Design review of the part built by this model. Coordinates are the model's own, in mm. Face numbers are marked on the shaded views. A direction names the side the tool comes from. Coordinates: 2 decimals unless noted, no trailing zeros. Loops run counter-clockwise (first coordinate to the right, second up) from the corner with the lowest first, then second, coordinate; pieces in that order, holes last. Notation, with made-up numbers: M -36,70 L -4,70 A21 cw -4,101 Z; hole C 28.25,-23 d3. An arc over 180 degrees is marked long. Answer as a JSON object with one key per item and string values. Group by question number.
1. Consider section C-C (y = 22). State the section outline as (x, z) points, then the cut area to 3 significant figures.
2. Consider section A-A (z = 0). State the section outline as (x, y) points, then the cut area to 3 significant figures.
3. To check wall thickness, follow probe 1 along Z at (x, y) = (-7, 5.5); probe 2 along X at (y, z) = (3, -2.5); probe 3 along X at (y, z) = (1.5, 0). State the ranges of each line that lie inside material, in increasing order.
4. Consider section B-B (x = 0). State the section outline as (y, z) points.
5. Insertion check: pin 1 (18 mm diameter, centred on x = -7.5, z = 3.5, fed in from +Y). The pin has a flat end and moves straight along its axis. Give the tip position at first contact, or say it passes through.
6. Draft analysis for pull direction X (two halves, no side actions). For the marked faces 3, 4, 5 and 6, state which applies: +X half, -X half, draft (parallel to the pull), parting line (faces both ways), or undercut.
7. Machinability: for the marked faces 1 and 2, which of the approach directions +Z, -Z, +X, -X, +Y, -Y give a long, thin tool a straight path to every point of the face, cutting with its end or side? Answer none if there is none.
8. Consider section D-D (z = -10.5). State the section outline as (x, y) points.
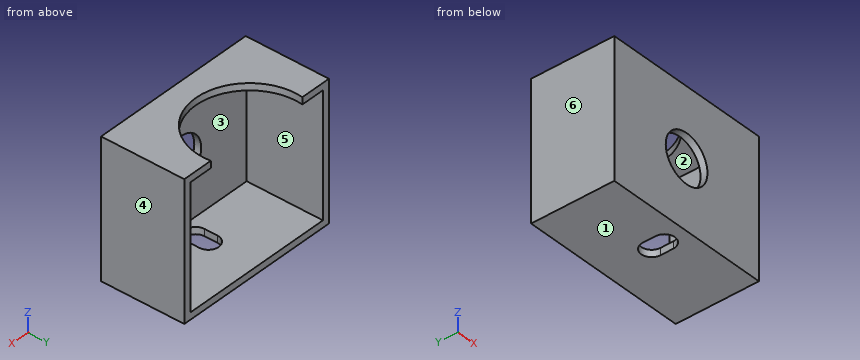
from build123d import *

# Parameters (mm, degrees)
SKETCH_2_W          = 48.5
SKETCH_2_H          = 39.5
EXTRUDE_1_DEPTH     = 2
SKETCH_4_W          = 48.5
SKETCH_4_H          = 39.5
SKETCH_4_W_2        = 44.5
SKETCH_4_H_2        = 35.5
EXTRUDE_2_DEPTH     = 22
SKETCH_5_R          = 15.5
CUT_EXTRUDE_1_DEPTH = 10
CUT_EXTRUDE_2_DEPTH = 10
SKETCH_7_R          = 7
CUT_EXTRUDE_3_DEPTH = 10


with BuildPart() as part:
    # 草图2 → 凸台-拉伸1 (new body)
    with BuildSketch(Plane(origin=(0, 0, 0), x_dir=(1, 0, 0), z_dir=(0, 1, 0))):
        Rectangle(SKETCH_2_W, SKETCH_2_H)
    extrude(amount=EXTRUDE_1_DEPTH)

    # 草图4 → 凸台-拉伸2 (add)
    with BuildSketch(Plane(origin=(0, 2, 0), x_dir=(1, 0, 0), z_dir=(0, 1, 0))):
        Rectangle(SKETCH_4_W, SKETCH_4_H)
        Rectangle(SKETCH_4_W_2, SKETCH_4_H_2, mode=Mode.SUBTRACT)
    extrude(amount=EXTRUDE_2_DEPTH)

    # 草图5 → 切除-拉伸1 (cut)
    with BuildSketch(Plane.XY.offset(19.75)):
        with Locations((0, 22)):
            Circle(SKETCH_5_R)
    extrude(amount=-CUT_EXTRUDE_1_DEPTH, mode=Mode.SUBTRACT)

    # 草图6 → 切除-拉伸2 (cut)
    with BuildSketch(Plane(origin=(0, 0, -19.75), x_dir=(-1, 0, 0), z_dir=(0, 0, -1))):
        with BuildLine():
            Line((3, 10.070876888), (3, 6.403632954))
            ThreePointArc((3, 6.403632954), (0, 3.403632954), (-3, 6.403632954))
            Line((-3, 6.403632954), (-3, 10.070876888))
            ThreePointArc((-3, 10.070876888), (0, 13.070876888), (3, 10.070876888))
        make_face()
    extrude(amount=-CUT_EXTRUDE_2_DEPTH, mode=Mode.SUBTRACT)

    # 草图7 → 切除-拉伸3 (cut)
    with BuildSketch(Plane.XZ):
        with Locations(Location((0, 0, 0), (0, 0, 270))):
            Circle(SKETCH_7_R)
    extrude(amount=-CUT_EXTRUDE_3_DEPTH, mode=Mode.SUBTRACT)


solid = part.part
Findings below:
{
 "1": {"outline": "M -24.25,-19.75 L 24.25,-19.75 L 24.25,19.75 L 15.5,19.75 L 15.5,17.75 L 22.25,17.75 L 22.25,-17.75 L -22.25,-17.75 L -22.25,17.75 L -15.5,17.75 L -15.5,19.75 L -24.25,19.75 Z", "area": "274 mm^2"},
 "2": {"outline": "M -24.25,0 L -7,0 L -7,2 L -22.25,2 L -22.25,24 L -24.25,24 Z; M 7,0 L 24.25,0 L 24.25,24 L 22.25,24 L 22.25,2 L 7,2 Z", "area": "157 mm^2"},
 "3": {"probe 1": "z = -19.75 to -17.75, 17.75 to 19.75", "probe 2": "x = -24.25 to -22.25, 22.25 to 24.25", "probe 3": "x = -24.25 to -7, 7 to 24.25"},
 "4": {"outline": "M 0,-19.75 L 3.4,-19.75 L 3.4,-17.75 L 2,-17.75 L 2,-7 L 0,-7 Z; M 0,7 L 2,7 L 2,17.75 L 6.5,17.75 L 6.5,19.75 L 0,19.75 Z; M 13.07,-19.75 L 24,-19.75 L 24,-17.75 L 13.07,-17.75 Z"},
 "5": {"pin 1": "stops at y = 2"},
 "6": {"face 3": "undercut", "face 4": "+X half", "face 5": "undercut", "face 6": "-X half"},
 "7": {"face 1": "-Z, +X, -X, +Y, -Y", "face 2": "+Y"},
 "8": {"outline": "M -24.25,0 L 24.25,0 L 24.25,24 L 22.25,24 L 22.25,2 L -22.25,2 L -22.25,24 L -24.25,24 Z"}
}
